Autodesk Inventor part; units mm, degrees
ref_plane "Work Plane1" through (0.2, -0.2, 2) normal (0, 0, -1) x (0, 1, 0)
ref_plane "YZ Plane" through (0, 0, 0) normal (1, 0, 0) x (0, 1, 0)
ref_plane "XZ Plane" through (0, 0, 0) normal (0, 1, 0) x (-1, 0, 0)
sketch "clip_sketch" plane through (0, 0, 0) normal (0, 0, 1) x (1, 0, 0)
  line L0 (0.2, -0.2) -> (9.8, -0.2)
  line L1 (9.8, -0.2) -> (9.8, 2.4)
  line L2 (0.2, 2.4) -> (9.8, 2.4)
  line L3 (0.2, -0.2) -> (0.2, 2.4)
  line L4 (0.4, -0.2) -> (0.4, 2.4)
  line L5 (9.6, 2.4) -> (9.6, -0.2)
  line L6 (0.4, -0.2) -> (0.4, -0.2)
  line L7 (-0.6, -1.2) -> (-0.6, -2.2)
  line L8 (3.4, -6.2) -> (6.6, -6.2)
  line L9 (10.6, -2.2) -> (10.6, -1.2)
  line L10 (9.6, -0.2) -> (9.6, -0.2)
  line L11 (0.4, 2.4) -> (0.4, 5.4)
  line L12 (0.4, 5.4) -> (9.6, 5.4)
  line L13 (9.6, 5.4) -> (9.6, 2.4)
  line L14 (3.4, -4) -> (2.4, 5.4)
  line L15 (6.6, -4) -> (7.6, 5.4)
  arc A0 (0.4, 5.4) -> (0.4, 2.4) centre (2.5, 3.9) ccw
  arc A1 (9.6, 2.4) -> (9.6, 5.4) centre (7.5, 3.9) ccw
  line L16 (5, 2.4) -> (5, -0.2) construction
  arc A2 (0.4, -0.2) -> (-0.6, -1.2) centre (0.4, -1.2) ccw
  arc A3 (10.6, -1.2) -> (9.6, -0.2) centre (9.6, -1.2) ccw
  arc A4 (-0.6, -2.2) -> (3.4, -6.2) centre (3.4, -2.2) ccw
  arc A5 (6.6, -6.2) -> (10.6, -2.2) centre (6.6, -2.2) ccw
  line L17 (3.4, -4) -> (6.6, -4)
  point P0 (0, 0)
  point P1 (-0.6, -0.2)
  dimension "d31" = 0.2
  dimension "d32" = 0.2
  dimension "d33" = 1
  dimension "d34" = 1
  dimension "d35" = 6
  dimension "d36" = 2
  dimension "d37" = 2
  dimension "d39" = 5
  dimension "d40" = 5
  dimension "d41" = 3
  dimension "d42" = 1
  dimension "d43" = 4
  dimension "d44" = 2.2
  dimension "d45" = 1
ref_plane "Work Plane1" through (0.2, -0.2, 2) normal (0, 0, -1) x (0, 1, 0)
extrude "clip" add sketch "clip_sketch" along normal blind 1.6 contours L4 L2 L14 L0 | L0 L14 L17 L15 A3 L9 A5 L8 A4 L7 A2 | L11 L12 L14 L2 | A0 L11 | L15 L2 L5 L0 | L15 L12 L13 L2 | L13 A1
fillet "teeth" radius 1 4 edges at (2.4, 5.4, 0.8) (7.6, 5.4, 0.8) (0.4, 5.4, 0.8) (9.6, 5.4, 0.8)
fillet "inside" radius 1.6 2 edges at (3.4, -4, 0.8) (6.6, -4, 0.8)
properties part number "fastener_lock" material "ABS Plastic"
Verification items for the finished model (mm, model axes). A direction names the side the tool comes from. Coordinates: 2 decimals unless noted, no trailing zeros. Order: outer loops, then holes, each group sorted by start corner. A loop starts at its lowest first (then second) coordinate and runs counter-clockwise, first axis right, second up. Notation, with made-up numbers: M 2,19.25 L 61,19.25 A12 cw 61,37.25 Z; hole C 16.5,-21.75 d1. An arc over 180 degrees is marked long. One line per item, written item: value. Start each with the question number.
Item 1: Sectioned sample at B-B on x = 9.75. Record the cut outline in (y, z).
Item 2: Sectioned sample at C-C on z = 1.3. Record the cut outline in (x, y), then the cut area to 3 significant figures.
Item 3: Sectioned sample at A-A on y = 3.25. Record the cut outline in (x, z).
Item 4: Access from +Z, -Z, +X, -X, +Y, -Y to the whole of each face (thin tool, end or side, straight path). Record for faces 1 (the flat face through (0.4, 1, 1)), 2 (the cylindrical face through (6.22, -3.6, 0.81)), 3 (the cylindrical face through (10.299, -0.485, 0.789)).
Item 5: Depth check by flat-ended pin: P1, Ø0.5, axis at y = 0.5, z = 0.5, coming from the -X side; P2, Ø1, axis at x = 8, y = -4.5, coming from the -Z side; P3, Ø0.8, axis at y = 1, z = 1, coming from the +X side. Enter the tip coordinate at first touch or a pass-through.
Item 6: Mould release check, pull along X, two halves, no side actions. Record for faces 4 (the flat face through (9.6, 1, 1)), 5 (the cylindrical face through (7.84, 5.15, 0.81)), 6 (the flat face through (-0.6, -2, 1)): pulls with the +X half, pulls with the -X half, needs draft (parallel to the pull), parting line crosses it, or undercut.
Item 7: Thickness scan on probe 1 along X at (y, z) = (2.25, 0.6); probe 2 along X at (y, z) = (-3.75, 0.8); probe 3 along X at (y, z) = (-4.25, 0.95). Record the ranges inside material, lowest first.
Item 8: Sectioned sample at D-D on x = 5.75. Record the cut outline in (y, z).
Calculated:
1. outline: M -4.67,0 L -0.21,0 L -0.21,1.6 L -4.67,1.6 Z; M 2.64,0 L 5.06,0 L 5.06,1.6 L 2.64,1.6 Z
2. outline: M -0.6,-2.2 A4 ccw 3.4,-6.2 L 6.6,-6.2 A4 ccw 10.6,-2.2 L 10.6,-1.2 A1 ccw 9.6,-0.2 L 9.6,2.4 A2.58 ccw 9.95,4.72 A1 ccw 9,5.4 L 8.5,5.4 A1 ccw 7.5,4.51 L 6.75,-2.57 A1.6 cw 5.16,-4 L 4.84,-4 A1.6 cw 3.25,-2.57 L 2.5,4.51 A1 ccw 1.5,5.4 L 1,5.4 A1 ccw 0.05,4.72 A2.58 ccw 0.4,2.4 L 0.4,-0.2 A1 ccw -0.6,-1.2 Z
2. area: 74.3 mm^2
3. outline: M 0,0 L 2.63,0 L 2.63,1.6 L 0,1.6 Z; M 7.37,0 L 10,0 L 10,1.6 L 7.37,1.6 Z
4. face 1: +Z, -Z, -X
4. face 2: +Z, -Z, +Y
4. face 3: +Z, -Z, +X
5. P1: x = 0.4
5. P2: z = 0
5. P3: x = 9.6
6. face 4: pulls with the +X half
6. face 5: undercut
6. face 6: pulls with the -X half
7. probe 1: 0.4 to 2.74, 7.26 to 9.6
7. probe 2: -0.29 to 3.98, 6.02 to 10.29
7. probe 3: -0.03 to 10.03
8. outline: M -6.2,0 L -3.89,0 L -3.89,1.6 L -6.2,1.6 Z
